Read the model definition and answer for the solid it produces. Units are mm, in the model's axes. A direction names the side the tool comes from. Give positions to 0.01 mm unless a question says otherwise; leave off trailing zeros. Loops run counter-clockwise (first coordinate to the right, second up) from the corner with the lowest first, then second, coordinate; pieces in that order, holes last. Notation, with made-up numbers: (48, -7.75) - (61, -7.75) arc R21 cw to (61, 28.25) - close; hole circle Ø6 at (-5, -12). An arc over 180 degrees is marked (long way). Write each question's results on one line, items separated by ' | '. Start each with the question number.
Q1. For faces 1 (the flat face through (-31.303, 21.129, 2.958)), 2 (the flat face through (-4.992, 11.553, 2.958)), 3 (the flat face through (-62, 23, 3)), determine the directions among +Z, -Z, +X, -X, +Y, -Y from which every point of the face is accessible in a straight line to the end or side of a thin tool.
Q2. Find the intervals of material crossed by line 1 (X direction, y = 7.25, z = 1.35); line 2 (X direction, y = 17.25, z = 1.7); line 3 (Y direction, x = -43, z = 4.1), in increasing order. Write a range as from..to.
Q3. Given pin 1 (1.3 mm diameter, centred on y = 8.5, z = 2.5, fed in from -X), flat-ended and moving along its own axis, determine where the tip first touches the part or whether it passes through.
Q4. The part is cut by section D-D, the plane x = -48. Write down the section's boundary in (y, z).
Q5. The part is cut by section B-B, the plane y = 28. Write down the section's boundary in (x, z), plus the area to 3 significant figures.
Q6. The part is cut by section C-C, the plane x = -7. Write down the section's boundary in (y, z).
Q7. Determine the mould class of faces 4 (the flat face through (-61, 18.5, 3)), 5 (the flat face through (-51.98, 28.65, 2.96)), 6 (the flat face through (0, 4, 3)), 7 (the flat face through (-32, 0, 3)) for opening direction Y: +Y half, -Y half, draft (parallel to the pull), parting line (faces both ways), or undercut.
```python
from build123d import *

# Parameters (mm, degrees)
ESQUISSE1_W        = 3
ESQUISSE1_H        = 7
BOSS_EXTRU_1_DEPTH = 6


with BuildPart() as part:
    # Esquisse1 → Boss.-Extru.1 (new body)
    with BuildSketch(Plane.XY):
        with Locations((-61.5, 26.5)):
            Rectangle(ESQUISSE1_W, ESQUISSE1_H)
        Polygon((-60, 15), (-60, 18.5), (-63, 18.5), (-63, 11.5), (-60, 11.5), align=None)
        with Locations((-61.5, 3.5)):
            Rectangle(ESQUISSE1_W, ESQUISSE1_H)
        Polygon((-52.482459034, 27.263838853), (-60, 30), (-60, 23), (-60, 18.5), (-60, 15), (-60, 11.5), (-60, 8.263368901), (-60, 7), (-60, 0), (0, 0), (0, 8.161785944), (-5.497827994, 10.162831687), (-13.015368961, 12.898992834), (-18.653524685, 14.951113694), (-26.171065652, 17.68727484), (-31.809221376, 19.7393957), (-39.326762343, 22.475556847), (-44.964918067, 24.527677707), align=None)
        Polygon((-51.48657782, 30), (-52.482459034, 27.263838853), (-44.964918067, 24.527677707), (-43.938857637, 27.346755569), (-51.2285868, 30), align=None)
        Polygon((-38.300701913, 25.294634709), (-39.326762343, 22.475556847), (-31.809221376, 19.7393957), (-30.783160946, 22.558473563), align=None)
        Polygon((-25.145005222, 20.506352703), (-26.171065652, 17.68727484), (-18.653524685, 14.951113694), (-17.627464255, 17.770191556), align=None)
        Polygon((-13.015368961, 12.898992834), (-5.497827994, 10.162831687), (-4.471767564, 12.981909549), (-11.989308531, 15.718070696), align=None)
    extrude(amount=BOSS_EXTRU_1_DEPTH)


solid = part.part
```
Check sheet entries:
1) face 1: +Z, -Z | face 2: +Z, -Z, +X | face 3: +Z, -Z, -X
2) line 1: x = -60..0 | line 2: x = -63..-17.82 | line 3: y = 0..23.81
3) pin 1: stops at x = -60
4) outline: (0, 0) - (28.82, 0) - (28.82, 6) - (0, 6) - close
5) outline: (-63, 0) - (-54.51, 0) - (-54.51, 6) - (-63, 6) - close; (-52.21, 0) - (-45.73, 0) - (-45.73, 6) - (-52.21, 6) - close | area: 89.9 mm^2
6) outline: (0, 0) - (13.9, 0) - (13.9, 6) - (0, 6) - close
7) face 4: undercut | face 5: +Y half | face 6: draft | face 7: -Y half
